Here's the drawing with two shaded views (mm, measured from the low corner). I have some questions. Coordinates: 2 decimals unless noted, no trailing zeros. Write each loop counter-clockwise with the first axis right and the second up, starting at its lowest first coordinate (ties: lowest second). Pieces come first, ordered by that corner, then holes. Notation, with made-up numbers: (45, 63) -> (58, 63) arc R19 ccw to (58, 75) -> close; hole circle Ø6 at (85, 12). An arc over 180 degrees is marked (long way). Put each result on its own line as item: value.
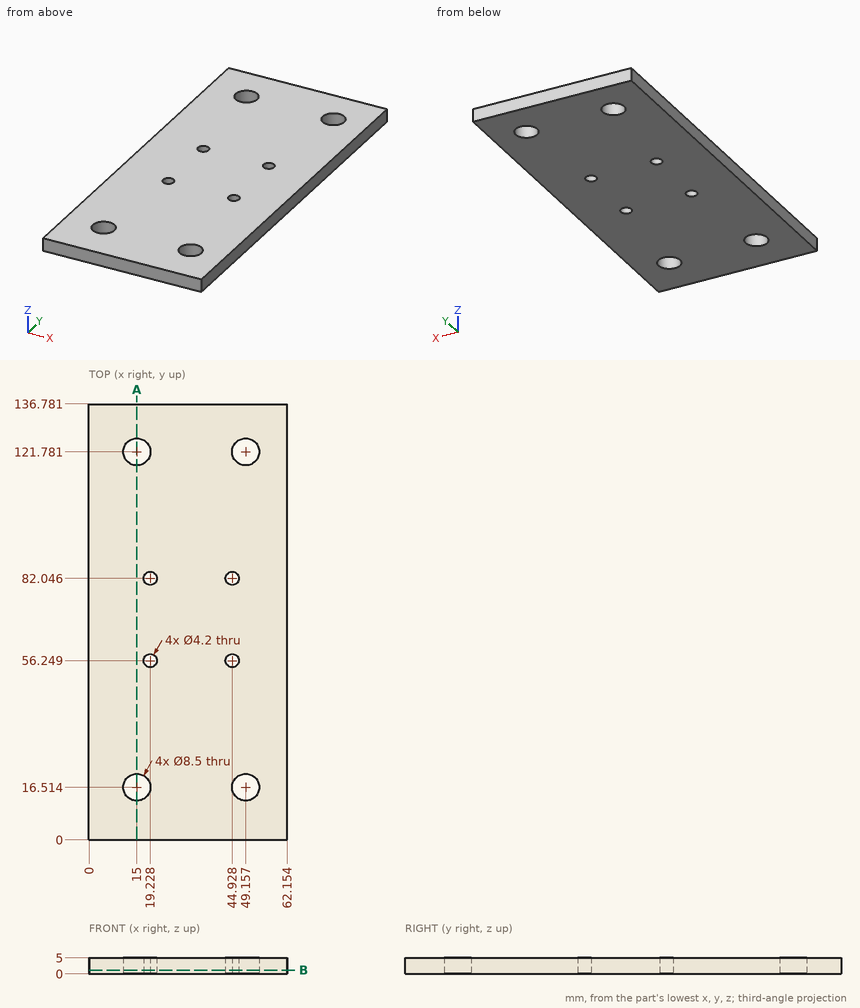
Item 1: Imagine slicing it at B-B on z = 1.2. State how many separate pieces and enclosed holes the cut face has, then the cut area to 3 significant figures.
Output:
separate pieces: 1
enclosed holes: 8
area: 8,220 mm²
Item 2: Imagine slicing it at A-A on x = 15. Write out the boundary of the cut face in (y, z) (1 decimal), then the cut area to 3 significant figures.
Output:
outline: (0, 0) -> (12.3, 0) -> (12.3, 5) -> (0, 5) -> close; (20.8, 0) -> (117.5, 0) -> (117.5, 5) -> (20.8, 5) -> close; (126, 0) -> (136.8, 0) -> (136.8, 5) -> (126, 5) -> close
area: 599 mm²
Item 3: Please list where these lines run through material, in increasing order: line 1 along Y through (x, z) = (15, 3.55) (1 decimal); line 2 along Y through (x, z) = (15.5, 3.45) (1 decimal); line 3 along X through (y, z) = (118.5, 0.6) (1 decimal). Write a range as from..to.
Output:
line 1: y = 0..12.3, 20.8..117.5, 126..136.8
line 2: y = 0..12.3, 20.7..117.6, 126..136.8
line 3: x = 0..12.3, 17.7..46.5, 51.9..62.2
Item 4: For P1, Ø3.5, axis at x = 19.23, y = 56.25, coming from the -Z side, with a flat end and sliding along its axis, tell me the tip position at first contact or that it passes through.
Output:
P1: passes through
